```python
from build123d import *

# Parameters (mm, degrees)
BOSS_EXTRUDE1_DEPTH = 3.175
SKETCH2_R           = 2.159
CUT_EXTRUDE1_DEPTH  = 159.781746826


with BuildPart() as part:
    # Sketch1 → Boss-Extrude1 (new body)
    with BuildSketch(Plane(origin=(0, 0, 0), x_dir=(1, 0, 0), z_dir=(0, 1, 0))):
        Polygon((-111.686526805, 95.25), (-127, 83.918625912), (-127, -83.918625912), (-111.686526805, -95.25), (111.686526805, -95.25), (127, -83.918625912), (127, 83.918625912), (111.686526805, 95.25), align=None)
        with BuildLine():
            Line((-107.95, -46.941679523), (-107.95, 46.941679523))
            ThreePointArc((-107.95, 46.941679523), (-106.983597986, 50.59457048), (-104.337251825, 53.291679523))
            Line((-104.337251825, 53.291679523), (-89.02377863, 64.62305361))
            ThreePointArc((-89.02377863, 64.62305361), (-79.714546423, 73.122295645), (-67.490526817, 76.2))
            Line((-67.490526817, 76.2), (67.490526817, 76.2))
            ThreePointArc((67.490526817, 76.2), (79.714546423, 73.122295645), (89.02377863, 64.62305361))
            Line((89.02377863, 64.62305361), (104.337251825, 53.291679523))
            ThreePointArc((104.337251825, 53.291679523), (106.983597986, 50.59457048), (107.95, 46.941679523))
            Line((107.95, 46.941679523), (107.95, -46.941679523))
            ThreePointArc((107.95, -46.941679523), (106.983597986, -50.59457048), (104.337251825, -53.291679523))
            Line((104.337251825, -53.291679523), (89.02377863, -64.62305361))
            ThreePointArc((89.02377863, -64.62305361), (79.714546423, -73.122295645), (67.490526817, -76.2))
            Line((67.490526817, -76.2), (-67.490526817, -76.2))
            ThreePointArc((-67.490526817, -76.2), (-79.714546423, -73.122295645), (-89.02377863, -64.62305361))
            Line((-89.02377863, -64.62305361), (-104.337251825, -53.291679523))
            ThreePointArc((-104.337251825, -53.291679523), (-106.983597986, -50.59457048), (-107.95, -46.941679523))
        make_face(mode=Mode.SUBTRACT)
    extrude(amount=BOSS_EXTRUDE1_DEPTH)

    # Sketch2 → Cut-Extrude1 (cut, through all)
    with BuildSketch(Plane(origin=(0, 3.175, 0), x_dir=(1, 0, 0), z_dir=(0, 1, 0))):
        with Locations(Location((-88.154790052, 79.46185563, 0), (0, 0, 270))):
            Circle(SKETCH2_R)
        with Locations(Location((88.154790052, 79.46185563, 0), (0, 0, 90))):
            Circle(SKETCH2_R)
        with Locations(Location((88.154790052, -79.46185563, 0), (0, 0, 270))):
            Circle(SKETCH2_R)
        with Locations(Location((-88.154790052, -79.46185563, 0), (0, 0, 90))):
            Circle(SKETCH2_R)
        with Locations(Location((-118.781736441, 56.799107455, 0), (0, 0, 90))):
            Circle(SKETCH2_R)
        with Locations(Location((118.781736441, 56.799107455, 0), (0, 0, 270))):
            Circle(SKETCH2_R)
        with Locations(Location((-118.781736441, -56.799107455, 0), (0, 0, 270))):
            Circle(SKETCH2_R)
        with Locations(Location((118.781736441, -56.799107455, 0), (0, 0, 90))):
            Circle(SKETCH2_R)
        with Locations(Location((0, -85.598, 0), (0, 0, 270))):
            Circle(SKETCH2_R)
        with Locations(Location((0, 85.598, 0), (0, 0, 90))):
            Circle(SKETCH2_R)
        with Locations(Location((-117.348, -0.020516524, 0), (0, 0, 270))):
            Circle(SKETCH2_R)
        with Locations(Location((117.348, -0.020516524, 0), (0, 0, 90))):
            Circle(SKETCH2_R)
    extrude(amount=-CUT_EXTRUDE1_DEPTH, mode=Mode.SUBTRACT)


solid = part.part
```
Part model, mm, in its own coordinate system. A direction names the side the tool comes from. Coordinates: 2 decimals unless noted, no trailing zeros. Order: outer loops, then holes, each group sorted by start corner. A loop starts at its lowest first (then second) coordinate and runs counter-clockwise, first axis right, second up. Notation, with made-up numbers: (0.25, -1.5) - (10.25, -1.5) arc R33 ccw to (10.25, 29.5) - close; hole circle Ø1 at (83.25, 49). An arc over 180 degrees is marked (long way). Return JSON: item names as keys, results as strings. Group by question number.
Item 1: Pin check, flat tip, straight feed: pin 1 (5 mm diameter, centred on x = 118.78, z = -56.8, fed in from +Y) (3 decimals). Stop position of the tip, or through.
Item 2: Pull direction Z, two halves, no side cores. Call faces 3 (the face through (119.45, 1.565, -89.505)), 4 (the face through (79.557, 1.565, -73.206)), 5 (the face through (119.24, 1.57, 89.66)): pulls with the +Z half, pulls with the -Z half, needs draft (parallel to the pull), parting line crosses it, or undercut.
Item 3: Cut at A-A (x = -32). List the corners of the cut face in (y, z) (3 decimals), plus the area to 3 significant figures.
Item 4: Cut at B-B (z = 34.5). List the corners of the cut face in (x, y) (3 decimals).
Item 5: Drill centre lines: probe 1 along Z at (x, y) = (-17, 1); probe 2 along X at (y, z) = (0.4, 18.5); probe 3 along X at (y, z) = (1.5, 55.5). Where is each one in solid material? Low to high. Write a range as from..to.
Item 6: Which spindle directions (+Z, -Z, +X, -X, +Y, -Y) get a long thin tool onto all of the face, cutting with end or side? Do faces 1 (the face through (-79.557, 1.565, 73.206)), 2 (the face through (-119.24, 1.57, -89.66)). Say none if no direction does.
Item 7: Cut at C-C (y = 1.25). State how many separate pieces and enclosed holes the cut face has, plus the area to 3 significant figures.
Check values:
{
 "1": {"pin 1": "stops at y = 3.175"},
 "2": {"face 3": "pulls with the -Z half", "face 4": "undercut", "face 5": "pulls with the +Z half"},
 "3": {"outline": "(0, -95.25) - (3.175, -95.25) - (3.175, -76.2) - (0, -76.2) - close; (0, 76.2) - (3.175, 76.2) - (3.175, 95.25) - (0, 95.25) - close", "area": "121 mm2"},
 "4": {"outline": "(-127, 0) - (-107.95, 0) - (-107.95, 3.175) - (-127, 3.175) - close; (107.95, 0) - (127, 0) - (127, 3.175) - (107.95, 3.175) - close"},
 "5": {"probe 1": "z = -95.25..-76.2, 76.2..95.25", "probe 2": "x = -127..-107.95, 107.95..127", "probe 3": "x = -127..-120.51, -117.06..-101.35, 101.35..117.06, 120.51..127"},
 "6": {"face 1": "+Y, -Y", "face 2": "-Z, -X, +Y, -Y"},
 "7": {"separate pieces": "1", "enclosed holes": "13", "area": "16,700 mm2"}
}
